Geometry check sheet. Reference: the model listing, model coordinates, mm. A direction names the side the tool comes from. Give positions to 0.01 mm unless a question says otherwise; leave off trailing zeros. Loops run counter-clockwise (first coordinate to the right, second up) from the corner with the lowest first, then second, coordinate; pieces in that order, holes last. Notation, with made-up numbers: (-2, -38.5) - (3, -38.5) arc R32 ccw to (3, -4.5) - close; hole circle Ø4 at (82.5, 88.25). An arc over 180 degrees is marked (long way). Use a Markdown table: item, result. Add a question column.
1. Cross-section at D-D on z = -69.85. Enter the section's corners in (x, y).
2. Material ranges on L1, parallel to X at y = 11.75, z = -6.35; L2, parallel to X at y = 32, z = -32.5; L3, parallel to X at y = 1.45, z = -69.85, recorded low to high.
3. Cross-section at A-A on x = 10.16. Count the separate pieces of the cut face and the enclosed holes in it, and give its area (3 significant figures).
4. Set-up check for faces 1 (the cylindrical face through (11.74, 10.47, -65.02)), 2 (the cylindrical face through (12.807, 6.803, -33.97)), 3 (the cylindrical face through (2.576, 12.192, -38.063)): record each of +Z, -Z, +X, -X, +Y, -Y from which the full face is reachable in a straight line by a thin tool's end or side.
5. Cross-section at C-C on y = 14.5. Enter the section's corners in (x, z).
6. Draft check along Z on faces 4 (the cylindrical face through (5.502, 16.153, -8.956)), 5 (the flat face through (5.08, 26, -38)), 6 (the cylindrical face through (2.58, 38.52, -31.69)), 7 (the flat face through (10, 0, -38)). Enter one of: pulls with the +Z half, pulls with the -Z half, needs draft (parallel to the pull), parting line crosses it, or undercut.
7. Depth check by flat-ended pin: P1, Ø2, axis at x = 16.5, y = 15, coming from the +Z side; P2, Ø8, axis at x = 6, y = 35.5, coming from the +Z side; P3, Ø5, axis at y = 32.5, z = -53, coming from the +X side. Enter the tip coordinate at first touch or a pass-through.
Autodesk Inventor part; units mm, degrees
ref_plane "YZ Plane" through (0, 0, 0) normal (1, 0, 0) x (0, 1, 0)
ref_plane "XZ Plane" through (0, 0, 0) normal (0, 1, 0) x (-1, 0, 0)
ref_plane "XY Plane" through (0, 0, 0) normal (0, 0, 1) x (1, 0, 0)
sketch "Sketch1" plane through (0, 0, 0) normal (0, 1, 0) x (-1, 0, 0)
  line L0 (0, 0) -> (-20.32, 0)
  line L1 (-20.32, 0) -> (-20.32, -76.2)
  line L2 (-20.32, -76.2) -> (0, -76.2)
  line L3 (0, -76.2) -> (0, 0)
  dimension "d0" = 20.32
  dimension "d1" = 76.2
extrude "Extrusion1" add sketch "Sketch1" along normal blind 7.62
sketch "Sketch2" plane through (0, 7.62, 0) normal (0, 1, 0) x (1, 0, 0)
  line L0 (0, 0) -> (0, 12.7)
  line L1 (0, 12.7) -> (20.32, 12.7)
  line L2 (20.32, 12.7) -> (20.32, 63.5)
  line L3 (20.32, 63.5) -> (0, 63.5)
  line L4 (0, 63.5) -> (0, 12.7)
  dimension "d4" = 12.7
  dimension "d5" = 20.32
  dimension "d6" = 50.8
extrude "Extrusion2" add sketch "Sketch2" along normal blind 43.18
sketch "Sketch3" plane through (20.32, 0, 0) normal (1, 0, 0) x (0, 0, -1)
  line L0 (12.7, 50.8) -> (63.5, 50.8)
  line L1 (38.1, 50.8) -> (38.1, 25.4)
  circle A0 centre (38.1, 25.4) radius 19.05
  point P0 (0, 0)
  dimension "d9" = 25.4
  dimension "d10" = 38.1
extrude "Extrusion3" cut sketch "Sketch3" against normal blind 15.24
fillet "Fillet1" radius 25.4 2 edges at (10.16, 50.8, -63.5) (10.16, 50.8, -12.7)
sketch "Sketch6" plane through (0, 7.62, 0) normal (0, 1, 0) x (1, 0, 0)
  line L0 (0, 0) -> (20.32, 0)
  line L1 (10.16, 0) -> (10.16, 6.35)
  line L2 (20.32, 76.2) -> (0, 76.2)
  line L3 (10.16, 76.2) -> (10.16, 69.85)
  dimension "d20" = 6.35
  dimension "d21" = 6.35
fillet "Fillet2" radius 25.4 2 edges at (10.16, 7.62, -63.5) (10.16, 7.62, -12.7)
hole "Hole1" at (10.16, 7.62, -6.35) at (10.16, 7.62, -69.85) direction (0, -1, 0) diameter 5.08 end through all counterbore diameter 10.16 counterbore depth 3.81
sketch "Sketch7" plane through (10.16, 7.62, -6.35) normal (0, -1, 0) x (1, 0, 0)
  circle A0 centre (0, 0) radius 5.08
  circle A1 centre (0, -63.5) radius 2.54
  line L0 (-2.54, -63.5) -> (0, -63.5)
  circle A2 centre (0, -63.5) radius 5.08
  point P0 (-10.16, 6.35)
  dimension "d30" = 10.16
  dimension "d31" = 10.16
extrude "Extrusion5" cut sketch "Sketch7" against normal blind 15.24 contours A0 | A1 | A2
sketch "Sketch9" plane through (5.08, 25.4, -38.1) normal (1, 0, 0) x (0, 0, -1)
  line L0 (0, 0) -> (0, -6.604)
  circle A0 centre (0, -6.604) radius 6.604
  line L1 (0, -6.604) -> (-3.302, -12.3232)
  line L2 (0, -6.604) -> (6.604, -6.604) construction
  line L3 (0, -6.604) -> (3.302, -12.3232)
  line L4 (0, -6.604) -> (6.604, -6.604) construction
  line L5 (-3.302, -12.3232) -> (-4.064, -13.6431)
  line L6 (3.302, -12.3232) -> (4.064, -13.6431)
  line L7 (3.302, -12.3232) -> (4.826, -12.3232) construction
  circle A1 centre (-4.064, -13.6431) radius 1.778
  circle A2 centre (4.064, -13.6431) radius 1.778
  circle A3 centre (0, 0) radius 19.05
  line L8 (-19.05, 0) -> (-17.526, 0)
  line L9 (-17.526, 0) -> (-15.875, 0)
  circle A4 centre (-15.875, 0) radius 1.651
  line L10 (19.05, 0) -> (17.526, 0)
  line L11 (17.526, 0) -> (15.875, 0)
  circle A5 centre (15.875, 0) radius 1.651
  line L12 (0, 0) -> (-9.525, 16.4978)
  line L13 (0, 0) -> (9.525, 16.4978)
  line L14 (-9.525, 16.4978) -> (-8.763, 15.178)
  line L15 (-8.763, 15.178) -> (-7.9375, 13.7482)
  line L16 (9.525, 16.4978) -> (8.763, 15.178)
  line L17 (8.763, 15.178) -> (7.9375, 13.7482)
  circle A6 centre (-7.9375, 13.7482) radius 1.651
  circle A7 centre (7.9375, 13.7482) radius 1.651
  point P0 (-38.1, -25.4)
  point P1 (-2.5627, -12.6905)
  point P2 (2.5627, -12.6905)
  point P3 (3.9897, -11.8666)
  point P4 (-3.9897, -11.8666)
  dimension "d47" = 6.604
  dimension "d48" = 120
  dimension "d49" = 60
  dimension "d50" = 1.524
  dimension "d51" = 1.524
  dimension "d52" = 60
  dimension "d53" = 3.556
  dimension "d54" = 3.556
  dimension "d55" = 1.524
  dimension "d56" = 1.651
  dimension "d57" = 1.524
  dimension "d58" = 1.651
  dimension "d59" = 1.524
  dimension "d60" = 1.651
  dimension "d61" = 1.524
  dimension "d62" = 1.651
extrude "Extrusion7" cut sketch "Sketch9" against normal blind 25.4 contours A0 A2 L3 L0 | L0 L1 A1 A0 | L3 A2 A0 A1 L1 | A1 L1 A0 | A0 A1 | A6 L12 | L12 A6 | A7 L13 | L13 A7 | A1 A0 L1 | A2 A0 L3 | L3 A0 A2 | A2 A0 | A4 | A5
properties part number "Motor Mount V2"
Values found:
| question | item | result |
|---|---|---|
| 1 | outline | (0, 0) - (7.62, 0) - (7.62, 3.81) - (5.08, 3.81) - (5.08, 12.72) - (0, 12.72) - close; (12.7, 0) - (20.32, 0) - (20.32, 12.72) - (15.24, 12.72) - (15.24, 3.81) - (12.7, 3.81) - close |
| 2 | L1 | x = 0 to 5.08, 15.24 to 20.32 |
| 2 | L2 | x = 0 to 5.08 |
| 2 | L3 | x = 0 to 7.62, 12.7 to 20.32 |
| 3 | separate pieces | 3 |
| 3 | enclosed holes | 1 |
| 3 | area | 1,280 mm2 |
| 4 | face 1 | +Y |
| 4 | face 2 | +X |
| 4 | face 3 | +X, -X |
| 5 | outline | (0, -68.38) - (5.3, -68.38) arc R5.08 cw to (15.02, -68.38) - (20.32, -68.38) - (20.32, -53.72) - (5.08, -53.72) - (5.08, -43.12) - (0, -43.12) - close; (0, -33.08) - (5.08, -33.08) - (5.08, -22.48) - (20.32, -22.48) - (20.32, -7.82) - (15.02, -7.82) arc R5.08 cw to (5.3, -7.82) - (0, -7.82) - close |
| 6 | face 4 | pulls with the +Z half |
| 6 | face 5 | undercut |
| 6 | face 6 | undercut |
| 6 | face 7 | needs draft |
| 7 | P1 | stops at z = -7.43 |
| 7 | P2 | stops at z = -13.44 |
| 7 | P3 | stops at x = 5.08 |
